For this review, take the finished solid that the model builds, in its own axes (mm). Face numbers are marked on the shaded views. A direction names the side the tool comes from. Give positions to 0.01 mm unless a question says otherwise; leave off trailing zeros. Loops run counter-clockwise (first coordinate to the right, second up) from the corner with the lowest first, then second, coordinate; pieces in that order, holes last. Notation, with made-up numbers: (12.25, 33.5) - (52.25, 33.5) arc R16 ccw to (52.25, 47.5) - close; hole circle Ø3 at (-17.5, 32.5). An arc over 180 degrees is marked (long way). Use CSV: the item, a comma, the result in double quotes. Start each with the question number.
1. Take a section at D-D on z = 1.75. Give the boundary of the cut face in (x, y), plus the area to 3 significant figures.
2. Mouldability with a two-part tool opening along X and no side actions: class the marked faces 4, 5 and 6 as pulls with the +X half, pulls with the -X half, needs draft (parallel to the pull), parting line crosses it, or undercut.
3. Wall thickness on line 1 (X direction, y = 7.5, z = 1.75); line 2 (Z direction, x = -6.75, y = 3.5); line 3 (Z direction, x = -1.5, y = 6.6): over which ranges is each line inside the solid? List them lowest first.
4. For the marked faces 1, 2 and 3, list the 3-axis set-ups (+Z, -Z, +X, -X, +Y, -Y) from which the entire face can be reached by the end or side of a thin tool; tool diameter is ignored.
5. Take a section at C-C on x = -3.75. Give the boundary of the cut face in (y, z).
6. Take a section at B-B on y = 2.75. Give the boundary of the cut face in (x, z), plus the area to 4 significant figures.
7. Take a section at A-A on z = 6. Give the boundary of the cut face in (x, y).
8. For pin 1 (0.7 mm diameter, centred on x = -2, z = 17.5, fed in from +Y); pin 2 (5 mm diameter, centred on x = -11.5, z = 13, fed in from +Y); pin 3 (4 mm diameter, centred on x = -11, z = 7, fed in from +Y), all flat-tipped, find the tip position at first contact; note any pin that passes through.
```python
from build123d import *

# Parameters (mm, degrees)
ESQUISSE3_W             = 28
ESQUISSE3_H             = 20
BOSS_EXTRU_1_DEPTH      = 8
ESQUISSE4_W             = 22
ESQUISSE4_H             = 14
ENL_V_MAT_EXTRU_1_DEPTH = 6
ESQUISSE5_W             = 22
ESQUISSE5_H             = 3
ENL_V_MAT_EXTRU_2_DEPTH = 4
ESQUISSE7_R             = 1
BOSS_EXTRU_2_DEPTH      = 5
ESQUISSE9_R             = 1.15
ENL_V_MAT_EXTRU_3_DEPTH = 2
ESQUISSE11_R            = 1.15
ENL_V_MAT_EXTRU_4_DEPTH = 2
ESQUISSE12_W            = 7
ESQUISSE12_H            = 6.5
BOSS_EXTRU_3_DEPTH      = 2


with BuildPart() as part:
    # Esquisse3 → Boss.-Extru.1 (new body)
    with BuildSketch(Plane(origin=(0, 0, 0), x_dir=(1, 0, 0), z_dir=(0, 1, 0))):
        with Locations((-14, -10)):
            Rectangle(ESQUISSE3_W, ESQUISSE3_H)
    extrude(amount=BOSS_EXTRU_1_DEPTH)

    # Esquisse4 → Enlèv. mat.-Extru.1 (cut)
    with BuildSketch(Plane(origin=(0, 8, 0), x_dir=(1, 0, 0), z_dir=(0, 1, 0))):
        with Locations((-14, -10)):
            Rectangle(ESQUISSE4_W, ESQUISSE4_H)
    extrude(amount=-ENL_V_MAT_EXTRU_1_DEPTH, mode=Mode.SUBTRACT)

    # Esquisse5 → Enlèv. mat.-Extru.2 (cut)
    with BuildSketch(Plane(origin=(0, 8, 0), x_dir=(1, 0, 0), z_dir=(0, 1, 0))):
        with Locations((-14, -18.5)):
            Rectangle(ESQUISSE5_W, ESQUISSE5_H)
    extrude(amount=-ENL_V_MAT_EXTRU_2_DEPTH, mode=Mode.SUBTRACT)

    # Esquisse7 → Boss.-Extru.2 (add)
    with BuildSketch(Plane(origin=(0, 2, 0), x_dir=(1, 0, 0), z_dir=(0, 1, 0))):
        with Locations(Location((-14, -6, 0), (0, 0, 270))):
            Circle(ESQUISSE7_R)
    extrude(amount=BOSS_EXTRU_2_DEPTH)

    # Esquisse9 → Enlèv. mat.-Extru.3 (cut)
    with BuildSketch(Plane(origin=(0, 8, 0), x_dir=(1, 0, 0), z_dir=(0, 1, 0))):
        with Locations(Location((-26.25, -1.75, 0), (0, 0, 270))):
            Circle(ESQUISSE9_R)
    enl_v_mat_extru_3 = extrude(amount=-ENL_V_MAT_EXTRU_3_DEPTH, mode=Mode.SUBTRACT)

    # Symétrie1: Enlèv. mat.-Extru.3 across plane
    add(enl_v_mat_extru_3.mirror(Plane.ZY.offset(14)), mode=Mode.SUBTRACT)

    # Esquisse11 → Enlèv. mat.-Extru.4 (cut)
    with BuildSketch(Plane(origin=(0, 8, 0), x_dir=(1, 0, 0), z_dir=(0, 1, 0))):
        with Locations(Location((-26.5, -17.5, 0), (0, 0, 270))):
            Circle(ESQUISSE11_R)
    enl_v_mat_extru_4 = extrude(amount=-ENL_V_MAT_EXTRU_4_DEPTH, mode=Mode.SUBTRACT)

    # Symétrie2: Enlèv. mat.-Extru.4 across plane
    add(enl_v_mat_extru_4.mirror(Plane.ZY.offset(14)), mode=Mode.SUBTRACT)

    # Esquisse12 → Boss.-Extru.3 (add)
    with BuildSketch(Plane(origin=(0, 2, 0), x_dir=(1, 0, 0), z_dir=(0, 1, 0))):
        with Locations((-14, -6.25)):
            Rectangle(ESQUISSE12_W, ESQUISSE12_H)
    extrude(amount=BOSS_EXTRU_3_DEPTH)


solid = part.part
```
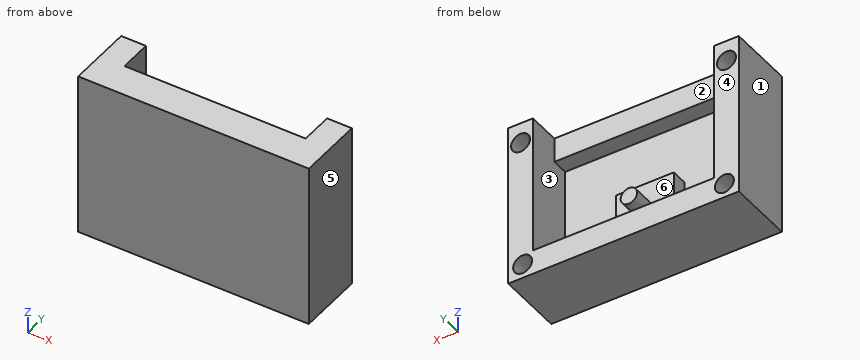
Check result:
1,outline,"(-28, 0) - (0, 0) - (0, 8) - (-0.6, 8) - (-0.6, 6) - (-2.9, 6) - (-2.9, 8) - (-25.1, 8) - (-25.1, 6) - (-27.4, 6) - (-27.4, 8) - (-28, 8) - close"
1,area,"215 mm²"
2,face 4,"needs draft"
2,face 5,"pulls with the +X half"
2,face 6,"undercut"
3,line 1,"x = -28 to -27.4, -25.1 to -2.9, -0.6 to 0"
3,line 2,"z = 0 to 3, 17 to 20"
3,line 3,"z = 0 to 0.63, 2.87 to 16.35, 18.65 to 20"
4,face 1,"+Z, -Z, -X, +Y, -Y"
4,face 2,"+Z, +Y"
4,face 3,"+Y"
5,outline,"(0, 0) - (8, 0) - (8, 3) - (2, 3) - (2, 17) - (4, 17) - (4, 20) - (0, 20) - close"
6,outline,"(-28, 0) - (0, 0) - (0, 20) - (-28, 20) - close; hole (-25, 3) - (-17.5, 3) - (-17.5, 9.5) - (-10.5, 9.5) - (-10.5, 3) - (-3, 3) - (-3, 17) - (-25, 17) - close"
6,area,"297.5 mm²"
7,outline,"(-28, 0) - (0, 0) - (0, 8) - (-3, 8) - (-3, 2) - (-10.5, 2) - (-10.5, 4) - (-13, 4) - (-13, 7) - (-15, 7) - (-15, 4) - (-17.5, 4) - (-17.5, 2) - (-25, 2) - (-25, 8) - (-28, 8) - close"
8,pin 1,"stops at y = 6"
8,pin 2,"stops at y = 2"
8,pin 3,"stops at y = 4"
